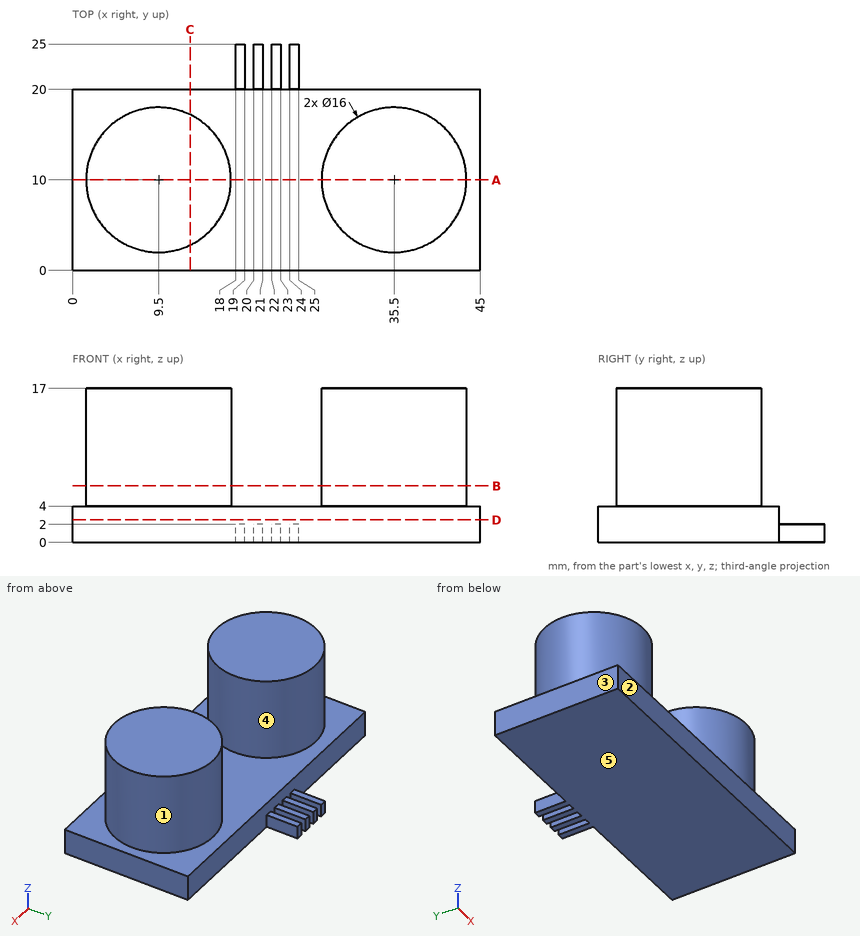
Study the drawing (mm; zero at the part's minimum x, y, z) and answer. A direction names the side the tool comes from. Coordinates: 2 decimals unless noted, no trailing zeros. Write each loop counter-clockwise with the first axis right and the second up, starting at its lowest first coordinate (ties: lowest second). Pieces come first, ordered by that corner, then holes. Notation, with made-up numbers: (-23, -5) - (16, -5) arc R24 ccw to (16, 16) - close; hole circle Ø6 at (-8, 19.5). An arc over 180 degrees is marked (long way). Put each result on its own line as item: value.
1. Find the intervals of material crossed by line 1 along Y through (x, z) = (18, 3); line 2 along X through (y, z) = (12.5, 9); line 3 along Z through (x, y) = (28, 5.5), in increasing order. Write a range as from..to.
Answer sheet:
line 1: y = 0..20
line 2: x = 1.9..17.1, 27.9..43.1
line 3: z = 0..4
2. The part is cut by section C-C on x = 13. Give the vertices of the cut face in (y, z), plus the area to 3 significant figures.
Answer sheet:
outline: (0, 0) - (20, 0) - (20, 4) - (17.19, 4) - (17.19, 17) - (2.81, 17) - (2.81, 4) - (0, 4) - close
area: 267 mm^2
3. A tool of negligible diameter and unlimited length cuts with its end or side. For the marked faces 1 and 2, from which of +Z, -Z, +X, -X, +Y, -Y can it reach the whole face along a straight path? Write none if from no direction.
Answer sheet:
face 1: +Z
face 2: +Z, -Z, +X, -X, -Y
4. The part is cut by section B-B on z = 6.25. Give the vertices of the cut face in (x, y).
Answer sheet:
outline: circle Ø16 at (9.5, 10); circle Ø16 at (35.5, 10)
5. Determine the mould class of the marked faces 3, 4 and 5 for opening direction X: pulls with the +X half, pulls with the -X half, needs draft (parallel to the pull), parting line crosses it, or undercut.
Answer sheet:
face 3: pulls with the -X half
face 4: undercut
face 5: needs draft
6. Flat-ended cylindrical pins translate along their axes: pin 1 Ø1.5 at (x, y) = (19.5, 14) entering from +Z; pin 2 Ø1.1 at (x, y) = (20.5, 22) entering from +Z; pin 3 Ø2 at (x, z) = (12.5, 3) entering from +Y. Find the tip coordinate at first contact, or state that the pin passes through.
Answer sheet:
pin 1: stops at z = 4
pin 2: stops at z = 2
pin 3: stops at y = 20
7. The part is cut by section D-D on z = 2.5. Give the vertices of the cut face in (x, y), plus the area to 3 significant figures.
Answer sheet:
outline: (0, 0) - (45, 0) - (45, 20) - (0, 20) - close
area: 900 mm^2
8. The part is cut by section A-A on y = 10. Give the vertices of the cut face in (x, z).
Answer sheet:
outline: (0, 0) - (45, 0) - (45, 4) - (43.5, 4) - (43.5, 17) - (27.5, 17) - (27.5, 4) - (17.5, 4) - (17.5, 17) - (1.5, 17) - (1.5, 4) - (0, 4) - close
